For this review, take the finished solid that the model builds, in its own axes (mm). A direction names the side the tool comes from. Coordinates: 2 decimals unless noted, no trailing zeros. Loops run counter-clockwise (first coordinate to the right, second up) from the corner with the lowest first, then second, coordinate; pieces in that order, holes last.
```python
from build123d import *

# Parameters (mm, degrees)
ESQUISSE1_R        = 1.5
BOSS_EXTRU_2_DEPTH = 6


with BuildPart() as part:
    # Esquisse1 → Boss.-Extru.2 (new body)
    with BuildSketch(Plane.XY):
        with BuildLine():
            Line((-9.65239237, 16.365552894), (-24.702558299, 24.270773037))
            Line((-24.702558299, 24.270773037), (-34.00281729, 6.564695473))
            Line((-34.00281729, 6.564695473), (-18.952651361, -1.34052467))
            ThreePointArc((-18.952651361, -1.34052467), (16.820773686, -8.835246042), (-9.65239237, 16.365552894))
        make_face()
        with Locations((-0.493805045, 13.991288596)):
            Circle(ESQUISSE1_R, mode=Mode.SUBTRACT)
        with Locations((12.363713879, -6.567996584)):
            Circle(ESQUISSE1_R, mode=Mode.SUBTRACT)
        with Locations((-11.869908833, -7.423292012)):
            Circle(ESQUISSE1_R, mode=Mode.SUBTRACT)
        with BuildLine():
            Line((-11.512444168, 12.824337382), (-23.021394585, 18.869505726))
            Line((-23.021394585, 18.869505726), (-28.601549979, 8.245859187))
            Line((-28.601549979, 8.245859187), (-17.092599563, 2.200690843))
            Line((-17.092599563, 2.200690843), (-13.988384403, 0.570176979))
            ThreePointArc((-13.988384403, 0.570176979), (-13.994675648, -0.386074479), (-13.935673418, -1.34052467))
            ThreePointArc((-13.935673418, -1.34052467), (-13.094244538, -3.227739126), (-11.285257604, -4.226311727))
            ThreePointArc((-11.285257604, -4.226311727), (-9.114394283, -5.700027795), (-8.739535981, -8.296942861))
            ThreePointArc((-8.739535981, -8.296942861), (-8.633495068, -10.360516531), (-7.304956633, -11.943098785))
            ThreePointArc((-7.304956633, -11.943098785), (0.493805045, -13.991288596), (8.128765127, -11.398384864))
            ThreePointArc((8.128765127, -11.398384864), (9.342426349, -9.72607885), (9.302722122, -7.66016391))
            ThreePointArc((9.302722122, -7.66016391), (9.493566014, -5.043283091), (11.555131282, -3.420188746))
            ThreePointArc((11.555131282, -3.420188746), (13.289218046, -2.296567787), (13.995505264, -0.354728625))
            ThreePointArc((13.995505264, -0.354728625), (11.869908833, 7.423292012), (5.806908291, 12.738909534))
            ThreePointArc((5.806908291, 12.738909534), (3.751818189, 12.953817976), (1.982535482, 11.886475637))
            ThreePointArc((1.982535482, 11.886475637), (-0.379171731, 10.743310886), (-2.815595301, 11.717131607))
            ThreePointArc((-2.815595301, 11.717131607), (-4.655722978, 12.657084318), (-6.690548632, 12.29782741))
            ThreePointArc((-6.690548632, 12.29782741), (-7.569542767, 11.777182273), (-8.408229009, 11.193823517))
            Line((-8.408229009, 11.193823517), (-11.512444168, 12.824337382))
        make_face(mode=Mode.SUBTRACT)
    extrude(amount=BOSS_EXTRU_2_DEPTH)


solid = part.part
```
Q1. Wall thickness on probe 1 along X at (y, z) = (-8.5, 2.4); probe 2 along Y at (x, z) = (-10.5, 3.3); probe 3 along X at (y, z) = (17, 1.45): over which ranges is each line inside the solid? List them lowest first.
Q2. Consider section A-A (z = 1.15). State the section outline as (x, y) points.
Q3. The part is to be moulded in two halves that separate along X. For faces 4 (the face through (-29.29, 15.54, 2.96)), 5 (the face through (-10, -5, 0)), 6 (the face through (11.173, -7.481, 2.958)), say which applies: +X half, -X half, draft (parallel to the pull), parting line (faces both ways), or undercut.
Q4. Consider section C-C (y = 17.5). State the section outline as (x, z) points, then the cut area to 3 significant figures.
Q5. Consider section D-D (x = 15). State the section outline as (y, z) points, then the cut area to 3 significant figures.
Q6. For pin 1 Ø6 at (x, y) = (-23, 4) entering from -Z; pin 2 Ø1.5 at (x, z) = (-18.5, 5) entering from +Y; pin 3 Ø8 at (x, y) = (-18.5, 7.5) entering from +Z; pin 4 Ø2 at (x, z) = (-18.5, 1) entering from +Y, all flat-tipped, find the tip position at first contact; note any pin that passes through.
Q7. Consider section B-B (x = -4). State the section outline as (y, z) points, then the cut area to 3 significant figures.
Q8. Machinability: for faces 1 (the face through (-25.772, 13.632, 2.958)), 2 (the face through (-17.07, 20.26, 2.96)), 3 (the face through (-26.583, 2.667, 2.958)), which of the approach directions +Z, -Z, +X, -X, +Y, -Y give a long, thin tool a straight path to every point of the face, cutting with its end or side? Answer none if there is none.
Model answer:
1. probe 1: x = -16.99 to -12.91, -10.83 to -8.79, 9.48 to 16.99
1. probe 2: y = -15.84 to -8.03, -6.81 to -4.48, 12.29 to 16.81
1. probe 3: x = -28.52 to -24, -19.46 to -10.86, -8.49 to 8.49
2. outline: (-34, 6.56) - (-18.95, -1.34) arc R19 ccw (long way) to (-9.65, 16.37) - (-24.7, 24.27) - close; hole (-28.6, 8.25) - (-13.99, 0.57) arc R14 ccw to (-13.94, -1.34) arc R3.25 ccw to (-11.29, -4.23) arc R3.25 cw to (-8.74, -8.3) arc R3.25 ccw to (-7.3, -11.94) arc R14 ccw to (8.13, -11.4) arc R3.25 ccw to (9.3, -7.66) arc R3.25 cw to (11.56, -3.42) arc R3.25 ccw to (14, -0.35) arc R14 ccw to (5.81, 12.74) arc R3.25 ccw to (1.98, 11.89) arc R3.25 cw to (-2.82, 11.72) arc R3.25 ccw to (-6.69, 12.3) arc R14 ccw to (-8.41, 11.19) - (-23.02, 18.87) - close; hole circle Ø3 at (-11.87, -7.42); hole circle Ø3 at (-0.49, 13.99); hole circle Ø3 at (12.36, -6.57)
3. face 4: -X half
3. face 5: draft
3. face 6: undercut
4. outline: (-28.26, 0) - (-23.74, 0) - (-23.74, 6) - (-28.26, 6) - close; (-20.41, 0) - (-11.81, 0) - (-11.81, 6) - (-20.41, 6) - close; (-7.4, 0) - (7.4, 0) - (7.4, 6) - (-7.4, 6) - close
4. area: 168 mm2
5. outline: (-11.66, 0) - (11.66, 0) - (11.66, 6) - (-11.66, 6) - close
5. area: 140 mm2
6. pin 1: stops at z = 0
6. pin 2: stops at y = 21.41
6. pin 3: passes through
6. pin 4: stops at y = 21.54
7. outline: (-18.57, 0) - (-13.42, 0) - (-13.42, 6) - (-18.57, 6) - close; (12.49, 0) - (18.57, 0) - (18.57, 6) - (12.49, 6) - close
7. area: 67.5 mm2
8. face 1: +Z, -Z
8. face 2: +Z, -Z, +Y
8. face 3: +Z, -Z, -X, -Y
